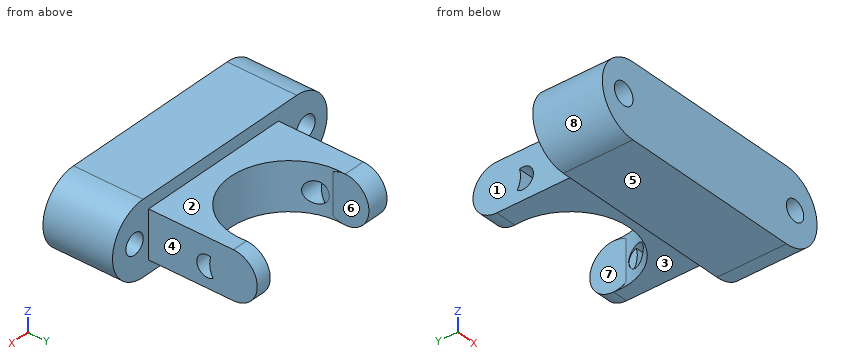
```python
from build123d import *

# Parameters (mm, degrees)
F0_W     = 66.5143355727
F0_H     = 26.5093380585
F1_DEPTH = 25.4
F2_R     = 4.014844692
F2_R_2   = 3.7572922796
F3_DEPTH = 25.4
F4_W     = 56.2347974628
F4_H     = 17.3515677452
F5_DEPTH = 30.988
F7_DEPTH = 32.512
F8_R     = 3.8559043701
F9_DEPTH = 79.502
F10_W    = 7.8387893736
F10_H    = 8.6757838726
F11_W    = 5.6234812364
F11_H    = 8.6757838726


with BuildPart() as f1:
    # F0 (on Front) → F1 (new body)
    with BuildSketch(Plane.XZ):
        with BuildLine():
            ThreePointArc((22.5329361856, -9.037273936), (35.7876052149, 4.2173950933), (22.5329361856, 17.4720641226))
            Line((22.5329361856, 17.4720641226), (22.5329361856, -9.037273936))
        make_face()
        with BuildLine():
            Line((-43.9813993871, -9.037273936), (-43.9813993871, 17.4720641226))
            ThreePointArc((-43.9813993871, 17.4720641226), (-57.2360684164, 4.2173950933), (-43.9813993871, -9.037273936))
        make_face()
        with Locations((-10.7242316008, 4.2173950933)):
            Rectangle(F0_W, F0_H)
    extrude(amount=F1_DEPTH)

    # F2 (on face) → F3 (cut)
    with BuildSketch(Plane.XZ.offset(25.4)):
        with Locations((-47.9707419872, 4.5908982866)):
            Circle(F2_R)
        with Locations((26.2565240264, 4.2173950933)):
            Circle(F2_R_2)
    extrude(amount=-F3_DEPTH, mode=Mode.SUBTRACT)

    # F4 (on face) → F5 (join)
    with BuildSketch(Plane(origin=(0, 0, 0), x_dir=(-1, 0, 0), z_dir=(0, 1, 0))):
        with Locations((7.9463692382, 4.2671263218)):
            Rectangle(F4_W, F4_H)
    extrude(amount=F5_DEPTH)

    # F6 (on face) → F7 (cut)
    with BuildSketch(Plane.XY.offset(12.9429101944)):
        with BuildLine():
            Line((14.5475482568, 30.988), (-28.224978596, 30.988))
            ThreePointArc((-28.224978596, 30.988), (-6.8387151696, 7.2567955588), (14.5475482568, 30.988))
        make_face()
    extrude(amount=-F7_DEPTH, mode=Mode.SUBTRACT)

    # F8 (on face) → F9 (cut)
    with BuildSketch(Plane(origin=(-36.0637679696, 0, 0), x_dir=(0, -1, 0), z_dir=(-1, 0, 0))):
        with Locations((-21.4650537819, 3.0787487049)):
            Circle(F8_R)
    extrude(amount=-F9_DEPTH, mode=Mode.SUBTRACT)

    # F10 (on face) → F12 (revolve)
    with BuildSketch(Plane(origin=(0, 30.988, 0), x_dir=(-1, 0, 0), z_dir=(0, 1, 0))):
        with Locations((32.1443732828, 8.6050182581)):
            Rectangle(F10_W, F10_H)
    revolve(axis=Axis((-32.1443732828, 30.988, 4.2671263218), (1, 0, 0)))

    # F11 (on face) → F13 (revolve)
    with BuildSketch(Plane(origin=(0, 30.988, 0), x_dir=(-1, 0, 0), z_dir=(0, 1, 0))):
        with Locations((-17.359288875, 8.6050182581)):
            Rectangle(F11_W, F11_H)
    revolve(axis=Axis((17.359288875, 30.988, 4.2671263218), (1, 0, 0)))


solid = f1.part
```
CAD build for the part. Positions are in the model's coordinates, mm. Face numbers are marked on the shaded views. A direction names the side the tool comes from. Give positions to 0.01 mm unless a question says otherwise; leave off trailing zeros. Order: outer loops, then holes, each group sorted by start corner. A loop starts at its lowest first (then second) coordinate and runs counter-clockwise, first axis right, second up.
(1) Tool access for the marked faces 1, 2, 3 and 4: list every direction of +Z, -Z, +X, -X, +Y, -Y with a clear straight run to the whole face (end or side of a thin tool).
(2) Saw through at D-D, the plane y = -17. Give the cut face in (x, z).
(3) Saw through at A-A, the plane x = 25.5. Give the cut face in (y, z).
(4) Saw through at C-C, the plane z = 10.5. Give the cut face in (x, y).
(5) Drill centre lines: L1, parallel to Z at x = -6.5, y = 5; L2, parallel to Y at x = -6, z = 13; L3, parallel to X at y = 33, z = 1. Where is each one in solid material? Low to high.
(6) Flat gauge pins, fed straight in: pin 1 (10 mm diameter, centred on y = 21.47, z = 3.08, fed in from -X); pin 2 (5 mm diameter, centred on y = 16, z = 10, fed in from +X); pin 3 (7 mm diameter, centred on x = -47.97, z = 4.59, fed in from +Y); pin 4 (25 mm diameter, centred on x = 3.5, y = 11.5, fed in from +Z). Where does each tip first touch, or does it go through?
(7) Saw through at B-B, the plane y = 35. Give the cut face in (x, z), then the cut area to 3 significant figures.
(8) Mould opens along X. For the marked faces 5, 6, 7 and 8 say: released by +X, released by -X, zero draft, split by the parting line, or undercut.
Results found:
1. face 1: +Z, -Z, -X, +Y
1. face 2: +Z, +X, -X, +Y
1. face 3: -Z, +X, -X, +Y
1. face 4: +Z, -Z, +X, +Y
2. outline: (-43.98, -9.04) - (22.53, -9.04) arc R13.25 ccw to (22.53, 17.47) - (-43.98, 17.47) arc R13.25 ccw to start; hole circle Ø8.03 at (-47.97, 4.59); hole circle Ø7.51 at (26.26, 4.22)
3. outline: (-25.4, -8.7) - (0, -8.7) - (0, 0.54) - (-25.4, 0.54) - close; (-25.4, 7.9) - (0, 7.9) - (0, 17.14) - (-25.4, 17.14) - close
4. outline: (-55.65, -25.4) - (34.2, -25.4) - (34.2, 0) - (20.17, 0) - (20.17, 37.02) - (14.55, 37.02) - (14.55, 26.53) arc R21.5 cw to (-28.22, 26.53) - (-28.22, 37.02) - (-36.06, 37.02) - (-36.06, 0) - (-55.65, 0) - close
5. L1: z = -4.41 to 12.94
5. L2: y = -25.4 to 0
5. L3: x = -36.06 to -28.22, 14.55 to 20.17
6. pin 1: stops at x = -36.06
6. pin 2: stops at x = 20.17
6. pin 3: passes through
6. pin 4: stops at z = 17.47
7. outline: (-36.06, -3.43) - (-28.22, -3.43) - (-28.22, 11.96) - (-36.06, 11.96) - close; (14.55, -3.43) - (20.17, -3.43) - (20.17, 11.96) - (14.55, 11.96) - close
7. area: 207 mm2
8. face 5: zero draft
8. face 6: undercut
8. face 7: undercut
8. face 8: released by -X
